Source: CAD feature listing. Evaluate the final solid. Frame: model axes, mm. A direction names the side the tool comes from. Round coordinates to 2 decimals unless told otherwise and drop trailing zeros. Loops run counter-clockwise (first coordinate to the right, second up) from the corner with the lowest first, then second, coordinate; pieces in that order, holes last. Notation, with made-up numbers: (65.5, 44.5) -> (121.5, 44.5) arc R24 cw to (121.5, 76.5) -> close; hole circle Ø9 at (51.5, -35). An arc over 180 degrees is marked (long way). Write item = value, one per line.
from build123d import *

# Parameters (mm, degrees)
EXTRUDE_1_DEPTH     = 20
SHELL_1_T           = -2
CUT_EXTRUDE_1_DEPTH = 100.679486355
FILLET_1_R          = 10
FILLET_2_R          = 3
SKETCH_3_W          = 50
SKETCH_3_H          = 52
EXTRUDE_2_DEPTH     = 2
SKETCH_4_R          = 10
EXTRUDE_3_DEPTH     = 10
SKETCH_5_R          = 1.5
CUT_EXTRUDE_2_DEPTH = 108.870292481
CUT_EXTRUDE_3_DEPTH = 100.19511746
CUT_EXTRUDE_4_REACH = 109.87
CUT_EXTRUDE_5_DEPTH = 108.870292481


with BuildPart() as part:
    # Sketch 1 → Extrude 1 (new, symmetric)
    with BuildSketch(Plane(origin=(0, 0, 0), x_dir=(1, 0, 0), z_dir=(0, 1, 0))):
        Polygon((42, -28), (-80, -28), (-80, 28), (42, 28), (80, 12.5), (80, -12.5), align=None)
    extrude(amount=EXTRUDE_1_DEPTH, both=True)

    # Shell 1
    shell_1_openings = [part.faces().sort_by_distance(p)[0] for p in [
        (-4.737705571, 20, 0),
        (-80, 0, 0),
        (-4.737705571, -20, 0),
    ]]
    offset(amount=SHELL_1_T, openings=shell_1_openings, kind=Kind.INTERSECTION)

    # Sketch 2 → Cut-Extrude 1 (cut, through all)
    with BuildSketch(Plane.XY.offset(28)):
        Polygon((-80, 12.5), (-78, 16.5), (-67.5, 20), (-80, 20), align=None)
        Polygon((-80, -12.5), (-78, -16.5), (-67.5, -20), (-80, -20), align=None)
        Polygon((-30, 20), (42, 11.25), (80, 11.25), (80, 20), align=None)
        Polygon((42, -11.25), (80, -11.25), (80, -20), (-30, -20), align=None)
    extrude(amount=-CUT_EXTRUDE_1_DEPTH, mode=Mode.SUBTRACT)

    # Fillet 1
    fillet_1_edges = [part.edges().sort_by_distance(p)[0] for p in [
        (41.607791612, 0, 26),
        (41.607791612, 0, -26),
    ]]
    fillet(fillet_1_edges, radius=FILLET_1_R)
    fillet_1_2_edges = [part.edges().sort_by_distance(p)[0] for p in [
        (42, 0, -28),
        (42, 0, 28),
    ]]
    fillet(fillet_1_2_edges, radius=FILLET_1_R)

    # Fillet 2
    fillet_2_edges = [part.edges().sort_by_distance(p)[0] for p in [
        (78, 0, -11.155809736),
        (78, 0, 11.155809736),
        (80, 0, -12.5),
        (80, 0, 12.5),
    ]]
    fillet(fillet_2_edges, radius=FILLET_2_R)

    # Sketch 3 → Extrude 2 (add)
    with BuildSketch(Plane(origin=(1.958559565, 16.116147275, 0), x_dir=(0.9926963020144297, -0.12064017559203144, 0), z_dir=(0.12064017559203145, 0.9926963020144298, 0))):
        with Locations((-7.193692572, 0)):
            Rectangle(SKETCH_3_W, SKETCH_3_H)
    extrude(amount=-EXTRUDE_2_DEPTH)

    # Sketch 4 → Extrude 3 (add)
    with BuildSketch(Plane(origin=(80, 0, 0), x_dir=(0, 0, -1), z_dir=(1, 0, 0))):
        with Locations(Location((0, 0, 0), (0, 0, 180))):
            Circle(SKETCH_4_R)
    extrude(amount=EXTRUDE_3_DEPTH)

    # Sketch 5 → Cut-Extrude 2 (cut, through all)
    with BuildSketch(Plane.XY.offset(28)):
        with Locations((-48, 0)):
            Circle(SKETCH_5_R)
    extrude(amount=-CUT_EXTRUDE_2_DEPTH, mode=Mode.SUBTRACT)

    # Sketch 6 → Cut-Extrude 3 (cut, through all)
    with BuildSketch(Plane(origin=(1.958559565, 16.116147275, 0), x_dir=(0.9926963020144297, -0.12064017559203144, 0), z_dir=(0.12064017559203145, 0.9926963020144298, 0))):
        Polygon((-18.193692572, -6), (-18.193692572, 6), (-12.193692572, 0), align=None)
        Polygon((-2.193692572, 2), (-17.193692572, 17), (-14.193692572, 17), (0.806307428, 2), align=None)
        Polygon((-14.193692572, -17), (0.806307428, -2), (-2.193692572, -2), (-17.193692572, -17), align=None)
    extrude(amount=-CUT_EXTRUDE_3_DEPTH, mode=Mode.SUBTRACT)

    # Sketch 7 → Cut-Extrude 4 (cut, up to next)
    with BuildSketch(Plane.XY.offset(28), mode=Mode.PRIVATE) as cut_extrude_4_sk1:
        with BuildLine():
            Line((-17.91886117, 2), (10, 2))
            Line((10, 2), (-16.131019724, 9.126641743))
            ThreePointArc((-16.131019724, 9.126641743), (-17.233482721, 9.002007909), (-17.94872078, 8.15383766))
            Line((-17.94872078, 8.15383766), (-19.341886117, 3.974341649))
            ThreePointArc((-19.341886117, 3.974341649), (-19.135724448, 2.622934573), (-17.91886117, 2))
        make_face()
    cut_extrude_4_tool1 = extrude(cut_extrude_4_sk1.sketch, amount=-CUT_EXTRUDE_4_REACH, mode=Mode.PRIVATE) & part.part
    # Sketch 7 → Cut-Extrude 4 (cut, up to next)
    with BuildSketch(Plane.XY.offset(28), mode=Mode.PRIVATE) as cut_extrude_4_sk2:
        with BuildLine():
            Line((-19.341886117, -3.974341649), (-17.94872078, -8.15383766))
            ThreePointArc((-17.94872078, -8.15383766), (-17.233482721, -9.002007909), (-16.131019724, -9.126641743))
            Line((-16.131019724, -9.126641743), (10, -2))
            Line((10, -2), (-17.91886117, -2))
            ThreePointArc((-17.91886117, -2), (-19.135724448, -2.622934573), (-19.341886117, -3.974341649))
        make_face()
    cut_extrude_4_tool2 = extrude(cut_extrude_4_sk2.sketch, amount=-CUT_EXTRUDE_4_REACH, mode=Mode.PRIVATE) & part.part
    cut_extrude_4_1 = cut_extrude_4_tool1.solids().sort_by_distance((-9.044619, 4.500562, 28))[0]
    add(cut_extrude_4_1, mode=Mode.SUBTRACT)
    cut_extrude_4_2 = cut_extrude_4_tool2.solids().sort_by_distance((-9.044619, -4.500562, 28))[0]
    add(cut_extrude_4_2, mode=Mode.SUBTRACT)
    cut_extrude_4 = cut_extrude_4_1 + cut_extrude_4_2  # Cut-Extrude 4 as one shape, for the pattern or mirror that repeats it

    # Mirror 1: Cut-Extrude 4 across plane
    add(cut_extrude_4.mirror(Plane.XY), mode=Mode.SUBTRACT)

    # Sketch 8 → Cut-Extrude 5 (cut, through all)
    with BuildSketch(Plane.XY.offset(28)):
        Polygon((-78, -6.25), (-78, 6.25), (-71.5, 8.727285854), (-68.173848955, 0), (-71.5, -8.727285854), align=None)
        Polygon((-66.414639843, 1), (-69.631129323, 9.43955153), (-66.272202597, 10.719708709), (-62.56781846, 1), align=None)
        Polygon((-66.272202597, -10.719708709), (-62.56781846, -1), (-66.414639843, -1), (-69.631129323, -9.43955153), align=None)
    extrude(amount=-CUT_EXTRUDE_5_DEPTH, mode=Mode.SUBTRACT)


solid = part.part
1. Section query C-C (x = 8). Return the cut outline in (y, z).
Evaluation:
outline = (-15.38, -28) -> (-2.55, -28) -> (-2.55, -26) -> (-15.38, -26) -> close; (-15.38, 26) -> (-2.55, 26) -> (-2.55, 28) -> (-15.38, 28) -> close; (-2, -28) -> (2, -28) -> (2, -26) -> (-2, -26) -> close; (-2, 26) -> (2, 26) -> (2, 28) -> (-2, 28) -> close; (2.55, -28) -> (15.38, -28) -> (15.38, 28) -> (2.55, 28) -> (2.55, 26) -> (13.37, 26) -> (13.37, -26) -> (2.55, -26) -> close
2. Line query: probe 1 along Z at (x, y) = (-32, 15.5); probe 2 along Y at (x, z) = (-48, -27.2); probe 3 along X at (y, z) = (-6.5, -9.5). Output: solid intervals per line, ascending. Write a range as from..to.
Evaluation:
probe_1 = -28..-26, 26..28
probe_2 = -20..-1.5, 1.5..20
probe_3 = 77.98..80
3. Mould query, pull axis Z, two halves, no side actions, for faces 4 (the face through (5.496, -15.686, 27.129)), 5 (the face through (60.73, 0.16, -20.36)), 6 (the face through (59.5, 0.2, -18.7)). Classes: released by +Z, released by -Z, zero draft, split by the parting line, or undercut.
Evaluation:
face_4 = zero draft
face_5 = released by -Z
face_6 = undercut
4. Contact query for flat-ended pins moving along their axis: pin 1 Ø3 at (x, y) = (58.5, -5.5) entering from +Z; pin 2 Ø1 at (x, z) = (-7, -27.5) entering from -Y; pin 3 Ø1 at (x, z) = (-6.5, 27) entering from +Y. Output: stop coordinate, or through.
Evaluation:
pin_1 = 21.88
pin_2 = -17.27
pin_3 = 17.2
5. Section query D-D (z = -22.5). Return the cut outline in (x, y).
Evaluation:
outline = (-30.24, 18.01) -> (19.39, 11.98) -> (19.63, 13.97) -> (-30, 20) -> close; (50.19, -11.25) -> (55.48, -11.25) -> (55.48, 11.25) -> (50.19, 11.25) -> close
6. Section query B-B (z = -15). Return the cut outline in (x, y), then the cut area to 3 significant figures.
Evaluation:
outline = (-30.24, 18.01) -> (-13.37, 15.96) -> (-13.12, 17.95) -> (-30, 20) -> close; (-10.39, 15.6) -> (19.39, 11.98) -> (19.63, 13.97) -> (-10.15, 17.59) -> close; (68.58, -11.25) -> (73.87, -11.25) -> (73.87, 11.25) -> (68.58, 11.25) -> close
area = 213 mm²
7. Section query A-A (x = -48). Return the cut outline in (y, z).
Evaluation:
outline = (-20, -28) -> (-1.5, -28) -> (-1.5, -26) -> (-20, -26) -> close; (-20, 26) -> (-1.5, 26) -> (-1.5, 28) -> (-20, 28) -> close; (1.5, -28) -> (20, -28) -> (20, -26) -> (1.5, -26) -> close; (1.5, 26) -> (20, 26) -> (20, 28) -> (1.5, 28) -> close
8. Set-up query: faces 1 (the face through (-72.824, -18.226, 27.014)), 2 (the face through (41.598, 0.162, 25.808)), 3 (the face through (-64.446, 5.928, 27.014)). Return all of +Z, -Z, +X, -X, +Y, -Y with unobstructed straight access to the full face (end or side cutting, diameter ignored); none if empty.
Evaluation:
face_1 = +Z, -Z, -X, -Y
face_2 = -X, +Y, -Y
face_3 = +Z, -Z
